Job drawing, mm, ordinate dimensions from the low corner. One solid piece. A direction names the side the tool comes from. Round coordinates to 2 decimals unless told otherwise and drop trailing zeros. Order: outer loops, then holes, each group sorted by start corner. A loop starts at its lowest first (then second) coordinate and runs counter-clockwise, first axis right, second up. Notation, with made-up numbers: (-13, 2.5) -> (32, 2.5) arc R35 cw to (32, 38.5) -> close; hole circle Ø9 at (46.5, 44.25). An arc over 180 degrees is marked (long way). Return JSON: item names as keys, results as strings. Group by question number.
Q1. Which spindle directions (+Z, -Z, +X, -X, +Y, -Y) get a long thin tool onto all of the face, cutting with end or side? Do the marked faces 4 and 5. Say none if no direction does.
Q2. Cut at B-B (y = 2.6). Write the cut outline in (x, z).
Q3. Probe line 1 along Y through (x, z) = (13, 7.75); line 2 along Y through (x, z) = (14.75, 3); line 3 along X through (y, z) = (17.8, 5.75). List the from-to ranges inside material, lowest first.
Q4. Cut at C-C (x = 8). Write the cut outline in (y, z).
Q5. Cut at A-A (z = 6.95). Write the cut outline in (x, y).
Q6. Cut at D-D (z = 1.5). Write the cut outline in (x, y).
Q7. Mould opens along Y. For the marked faces 1, 2 and 3 say: +Y half, -Y half, draft (parallel to the pull), parting line (faces both ways), or undercut.
Q8. Flat gauge pin, fed straight in: pin 1 (5 mm diameter, centred on y = 11.5, z = 7.5, fed in from -X). Where does the tip first touch, or does it go through?
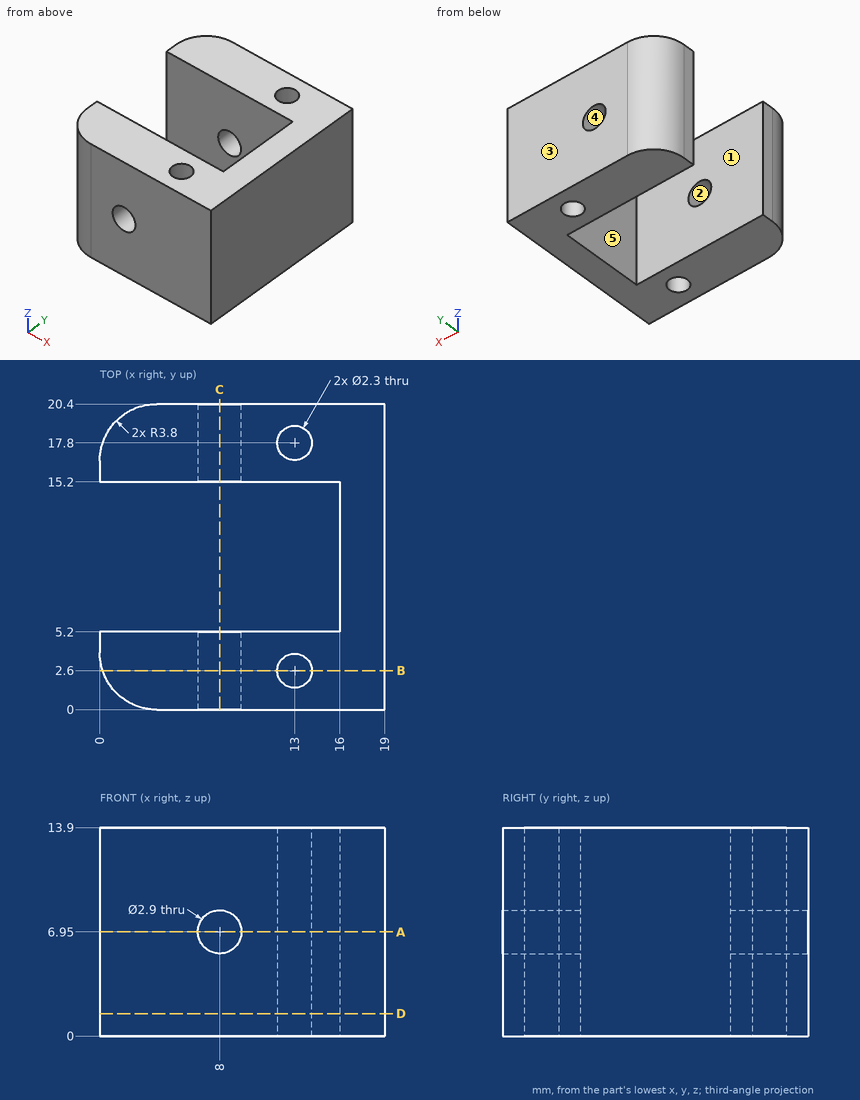
Solution:
{
 "1": {"face 4": "+Y, -Y", "face 5": "+Z, -Z, -X"},
 "2": {"outline": "(0.19, 0) -> (11.85, 0) -> (11.85, 13.9) -> (0.19, 13.9) -> close; (14.15, 0) -> (19, 0) -> (19, 13.9) -> (14.15, 13.9) -> close; hole circle Ø2.9 at (8, 6.95)"},
 "3": {"line 1": "y = 0 to 1.45, 3.75 to 5.2, 15.2 to 16.65, 18.95 to 20.4", "line 2": "y = 0 to 5.2, 15.2 to 20.4", "line 3": "x = 0.19 to 7.19, 8.81 to 11.85, 14.15 to 19"},
 "4": {"outline": "(0, 0) -> (5.2, 0) -> (5.2, 5.5) -> (0, 5.5) -> close; (0, 8.4) -> (5.2, 8.4) -> (5.2, 13.9) -> (0, 13.9) -> close; (15.2, 0) -> (20.4, 0) -> (20.4, 5.5) -> (15.2, 5.5) -> close; (15.2, 8.4) -> (20.4, 8.4) -> (20.4, 13.9) -> (15.2, 13.9) -> close"},
 "5": {"outline": "(0, 3.8) arc R3.8 ccw to (3.8, 0) -> (6.55, 0) -> (6.55, 5.2) -> (0, 5.2) -> close; (0, 15.2) -> (6.55, 15.2) -> (6.55, 20.4) -> (3.8, 20.4) arc R3.8 ccw to (0, 16.6) -> close; (9.45, 0) -> (19, 0) -> (19, 20.4) -> (9.45, 20.4) -> (9.45, 15.2) -> (16, 15.2) -> (16, 5.2) -> (9.45, 5.2) -> close; hole circle Ø2.3 at (13, 2.6); hole circle Ø2.3 at (13, 17.8)"},
 "6": {"outline": "(0, 3.8) arc R3.8 ccw to (3.8, 0) -> (19, 0) -> (19, 20.4) -> (3.8, 20.4) arc R3.8 ccw to (0, 16.6) -> (0, 15.2) -> (16, 15.2) -> (16, 5.2) -> (0, 5.2) -> close; hole circle Ø2.3 at (13, 2.6); hole circle Ø2.3 at (13, 17.8)"},
 "7": {"face 1": "undercut", "face 2": "draft", "face 3": "+Y half"},
 "8": {"pin 1": "stops at x = 16"}
}
